```python
from build123d import *

# Parameters (mm, degrees)
EXTRUDE_1_DEPTH     = 57.7
EXTRUDE_2_DEPTH     = 30.8
SKETCH_5_R          = 4
CUT_EXTRUDE_1_DEPTH = 15
SKETCH_7_W          = 6
SKETCH_7_H          = 7
SKETCH_7_R          = 2
EXTRUDE_3_DEPTH     = 2
SKETCH_8_W          = 6
SKETCH_8_H          = 1.5
EXTRUDE_4_DEPTH     = 6
EXTRUDE_START       = -37
SKETCH_8_3_W        = 6
SKETCH_8_3_H        = 1.5
EXTRUDE_5_DEPTH     = 6
SKETCH_9_R          = 2
CUT_EXTRUDE_2_DEPTH = 6
SKETCH_10_R         = 13
CUT_EXTRUDE_3_DEPTH = 49.696406438


with BuildPart() as part:
    # 스케치1 → 보스-돌출1 (new body)
    with BuildSketch(Plane.XY):
        with BuildLine():
            Line((-13.5, 0), (-18.5, 0))
            Line((-18.5, 0), (-18.5, -18.5))
            Line((-18.5, -18.5), (18.5, -18.5))
            Line((18.5, -18.5), (18.5, 0))
            Line((18.5, 0), (13.5, 0))
            ThreePointArc((13.5, 0), (0, -13.5), (-13.5, 0))
        make_face()
    extrude(amount=-EXTRUDE_1_DEPTH)

    # 스케치3 → 보스-돌출2 (add)
    with BuildSketch(Plane.XY.offset(-26.9)):
        with BuildLine():
            Line((-13.5, 0), (-11.5, 0))
            ThreePointArc((-11.5, 0), (0, -11.5), (11.5, 0))
            Line((11.5, 0), (13.5, 0))
            ThreePointArc((13.5, 0), (0, -13.5), (-13.5, 0))
        make_face()
    extrude(amount=-EXTRUDE_2_DEPTH)

    # 스케치5 → 컷-돌출1 (cut)
    with BuildSketch(Plane.ZY.offset(-18.5)):
        with Locations((-21.9, 0)):
            Circle(SKETCH_5_R)
    extrude(amount=CUT_EXTRUDE_1_DEPTH, mode=Mode.SUBTRACT)

    # 스케치7 → 보스-돌출3 (add)
    # profile 1 of 2: a face of its own
    with BuildSketch(Plane.XZ.offset(18.5)):
        with Locations((6.5, 3.5)):
            Rectangle(SKETCH_7_W, SKETCH_7_H)
        with Locations(Location((6.5, 4.15, 0), (0, 0, 270))):
            Circle(SKETCH_7_R, mode=Mode.SUBTRACT)
    # profile 2 of 2: a face of its own
    with BuildSketch(Plane.XZ.offset(18.5)):
        with Locations((-12.5, 3.5)):
            Rectangle(SKETCH_7_W, SKETCH_7_H)
        with Locations(Location((-12.5, 4.15, 0), (0, 0, 270))):
            Circle(SKETCH_7_R, mode=Mode.SUBTRACT)
    extrude_3 = extrude(amount=-EXTRUDE_3_DEPTH)

    # 대칭 복사1: 보스-돌출3 across plane
    add(extrude_3.mirror(Plane.XY.offset(-28.85)))

    # 스케치8 → 보스-돌출4 (add)
    with BuildSketch(Plane.ZY.offset(18.5)):
        with Locations((-9, -0.75)):
            Rectangle(SKETCH_8_W, SKETCH_8_H)
        with Locations((-37.7, -0.75)):
            Rectangle(SKETCH_8_W, SKETCH_8_H)
    extrude(amount=EXTRUDE_4_DEPTH)

    # 스케치8<3> → 보스-돌출5 (add)
    with BuildSketch(Plane.ZY.offset(18.5).offset(EXTRUDE_START)):
        with Locations((-9, -0.75)):
            Rectangle(SKETCH_8_3_W, SKETCH_8_3_H)
        with Locations((-37.7, -0.75)):
            Rectangle(SKETCH_8_3_W, SKETCH_8_3_H)
    extrude(amount=-EXTRUDE_5_DEPTH)

    # 스케치9 → 컷-돌출2 (cut)
    with BuildSketch(Plane(origin=(0, 0, 0), x_dir=(1, 0, 0), z_dir=(0, 1, 0))):
        with Locations(Location((-21.5, 37.7, 0), (0, 0, 180))):
            Circle(SKETCH_9_R)
        with Locations(Location((-21.5, 9, 0), (0, 0, 180))):
            Circle(SKETCH_9_R)
        with Locations(Location((21.5, 9, 0), (0, 0, 180))):
            Circle(SKETCH_9_R)
        with Locations(Location((21.5, 37.7, 0), (0, 0, 90))):
            Circle(SKETCH_9_R)
    extrude(amount=-CUT_EXTRUDE_2_DEPTH, mode=Mode.SUBTRACT)

    # 스케치10 → 컷-돌출3 (cut, through all)
    with BuildSketch(Plane.XY.offset(-26.9)):
        Circle(SKETCH_10_R)
    extrude(amount=-CUT_EXTRUDE_3_DEPTH, mode=Mode.SUBTRACT)


solid = part.part
```
For this review, take the finished solid that the model builds, in its own axes (mm). A direction names the side the tool comes from. Round coordinates to 2 decimals unless told otherwise and drop trailing zeros. Write each loop counter-clockwise with the first axis right and the second up, starting at its lowest first coordinate (ties: lowest second). Pieces come first, ordered by that corner, then holes. Notation, with made-up numbers: (89.5, 4.25) - (138.5, 4.25) arc R9 cw to (138.5, 12.25) - close; hole circle Ø9 at (78, -3.75). An arc over 180 degrees is marked (long way). Use CSV: the item, a comma, the result in double quotes.
1) Wall thickness on line 1 along Z through (x, y) = (-21.5, -1.15); line 2 along X through (y, z) = (-8.5, -27.5); line 3 along Z through (x, y) = (-5, -14): over which ranges is each line inside the solid? List them lowest first. Write a range as from..to.
Conclusion:
line 1,"z = -40.7..-39.7, -35.7..-34.7, -12..-11, -7..-6"
line 2,"x = -18.5..-9.84, 9.84..18.5"
line 3,"z = -57.7..0"
2) For faces 1 (the flat face through (21, -1, -12)), 2 (the flat face through (-19, -1.5, -9)), 3 (the flat face through (6, -16.5, 2)), list the 3-axis set-ups (+Z, -Z, +X, -X, +Y, -Y) from which the entire face can be reached by the end or side of a thin tool; tool diameter is ignored.
Conclusion:
face 1,"+X, +Y, -Y"
face 2,"+Z, -Z, -X, -Y"
face 3,"+Z, +X, -X, +Y"
3) Clearance check with flat-ended pins moving along their axes: pin 1 Ø1.5 at (y, z) = (-3, -28) entering from -X; pin 2 Ø2.5 at (x, z) = (21.5, -9) entering from -Y; pin 3 Ø0.8 at (x, y) = (-21.5, -0.5) entering from -Z; pin 4 Ø1 at (y, z) = (-17.5, 5) entering from -X. State where each tip first meets the part, or that it passes through.
Conclusion:
pin 1,"stops at x = -18.5"
pin 2,"passes through"
pin 3,"stops at z = -40.7"
pin 4,"stops at x = -15.5"
4) Add section D-D on y = -11.25. Write out the cut boundary in (x, z).
Conclusion:
outline,"(-18.5, -57.7) - (-6.51, -57.7) - (-6.51, -26.9) - (-7.46, -26.9) - (-7.46, 0) - (-18.5, 0) - close; (6.51, -57.7) - (18.5, -57.7) - (18.5, 0) - (7.46, 0) - (7.46, -26.9) - (6.51, -26.9) - close"
5) The part is to be moulded in two halves that separate along X. For faces 4 (the flat face through (21, -1, -40.7)), 5 (the flat face through (-15.5, -18, -61)), 6 (the cylindrical face through (0, -13, -42)), say which applies: pulls with the +X half, pulls with the -X half, needs draft (parallel to the pull), parting line crosses it, or undercut.
Conclusion:
face 4,"needs draft"
face 5,"pulls with the -X half"
face 6,"undercut"
6) Add section B-B on z = -9. Write out the cut boundary in (x, y), and give its area (3 significant figures).
Conclusion:
outline,"(-24.5, -1.5) - (-23.5, -1.5) - (-23.5, 0) - (-24.5, 0) - close; (-19.5, -1.5) - (-18.5, -1.5) - (-18.5, -18.5) - (18.5, -18.5) - (18.5, -1.5) - (19.5, -1.5) - (19.5, 0) - (13.5, 0) arc R13.5 cw to (-13.5, 0) - (-19.5, 0) - close; (23.5, -1.5) - (24.5, -1.5) - (24.5, 0) - (23.5, 0) - close"
area,"404 mm^2"
7) Add section C-C on y = -3.25. Write out the cut boundary in (x, z), and give its area (3 significant figures).
Conclusion:
outline,"(-18.5, -57.7) - (-12.59, -57.7) - (-12.59, -26.9) - (-13.1, -26.9) - (-13.1, 0) - (-18.5, 0) - close; (12.59, -57.7) - (18.5, -57.7) - (18.5, -24.23) - (13.1, -24.23) - (13.1, -26.9) - (12.59, -26.9) - close; (13.1, -19.57) - (18.5, -19.57) - (18.5, 0) - (13.1, 0) - close"
area,"629 mm^2"
8) Add section A-A on z = 4.15. Write out the cut boundary in (x, y).
Conclusion:
outline,"(-15.5, -18.5) - (-14.5, -18.5) - (-14.5, -16.5) - (-15.5, -16.5) - close; (-10.5, -18.5) - (-9.5, -18.5) - (-9.5, -16.5) - (-10.5, -16.5) - close; (3.5, -18.5) - (4.5, -18.5) - (4.5, -16.5) - (3.5, -16.5) - close; (8.5, -18.5) - (9.5, -18.5) - (9.5, -16.5) - (8.5, -16.5) - close"
